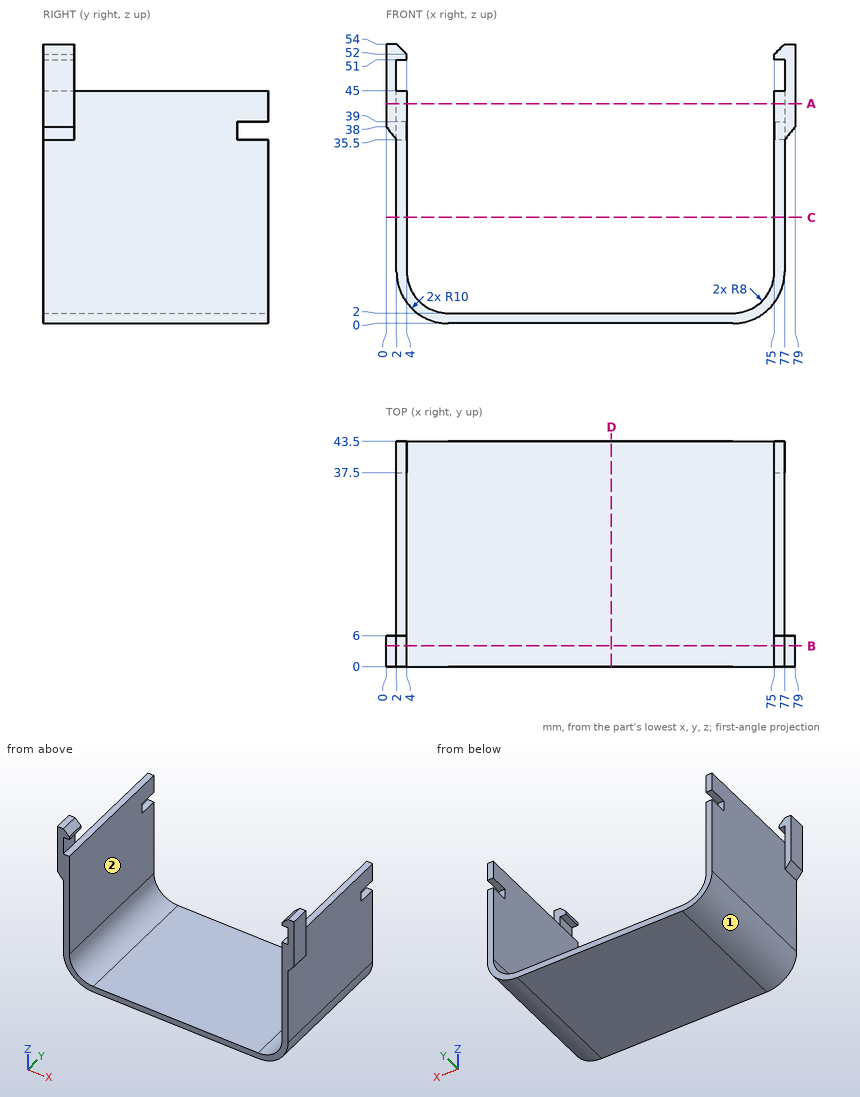
Job drawing, mm, ordinate dimensions from the low corner. One solid piece. A direction names the side the tool comes from. Round coordinates to 2 decimals unless told otherwise and drop trailing zeros. Write each loop counter-clockwise with the first axis right and the second up, starting at its lowest first coordinate (ties: lowest second). Pieces come first, ordered by that corner, then holes. Notation, with made-up numbers: M -26,15 L 20,15 A20 ccw 20,25 Z; hole C 11.25,-22 d3. An arc over 180 degrees is marked long. Return JSON: item names as keys, results as strings. Group by question number.
(1) Which spindle directions (+Z, -Z, +X, -X, +Y, -Y) get a long thin tool onto all of the face, cutting with end or side? Do the marked faces 1 and 2. Say none if no direction does.
(2) Saw through at D-D on x = 43.5. Write the cut outline in (y, z), then the cut area to 3 significant figures.
(3) Saw through at C-C on z = 20.5. Write the cut outline in (x, y), then the cut area to 3 significant figures.
(4) Saw through at A-A on z = 42.5. Write the cut outline in (x, y), then the cut area to 3 significant figures.
(5) Pin check, flat tips, straight feed: pin 1 Ø1 at (x, y) = (76, 39.5) entering from +Z; pin 2 Ø1.6 at (x, z) = (3, 37.5) entering from +Y; pin 3 Ø1 at (x, y) = (3.5, 42) entering from -Z. Stop position of each tip, or through.
(6) Drill centre lines: probe 1 along X at (y, z) = (8, 40); probe 2 along Z at (x, y) = (42, 5); probe 3 along X at (y, z) = (40.5, 3). Where is each one in solid material? Low to high.
(7) Saw through at B-B on y = 4. Write the cut outline in (x, z), then the cut area to 3 significant figures.
Returned:
{
 "1": {"face 1": "-Z, -X, +Y, -Y", "face 2": "+Z, +Y, -Y"},
 "2": {"outline": "M 0,0 L 43.5,0 L 43.5,2 L 0,2 Z", "area": "87.0 mm²"},
 "3": {"outline": "M 2,0 L 4,0 L 4,43.5 L 2,43.5 Z; M 75,0 L 77,0 L 77,43.5 L 75,43.5 Z", "area": "174 mm²"},
 "4": {"outline": "M 0,0 L 4,0 L 4,43.5 L 2,43.5 L 2,6 L 0,6 Z; M 75,0 L 79,0 L 79,6 L 77,6 L 77,43.5 L 75,43.5 Z", "area": "198 mm²"},
 "5": {"pin 1": "z = 45", "pin 2": "y = 37.5", "pin 3": "z = 4"},
 "6": {"probe 1": "2 to 4, 75 to 77", "probe 2": "0 to 2", "probe 3": "4.86 to 8.13, 70.87 to 74.14"},
 "7": {"outline": "M 0,38 L 2,35.5 L 2,10 A10 ccw 12,0 L 67,0 A10 ccw 77,10 L 77,35.5 L 79,38 L 79,54 L 77,54 L 75,52 L 75,51 L 77,51 L 77,45 L 75,45 L 75,10 A8 cw 67,2 L 12,2 A8 cw 4,10 L 4,45 L 2,45 L 2,51 L 4,51 L 4,52 L 2,54 L 0,54 Z", "area": "384 mm²"}
}
